Part model, mm, in its own coordinate system. Give positions to 0.01 mm unless a question says otherwise; leave off trailing zeros. Write each loop counter-clockwise with the first axis right and the second up, starting at its lowest first coordinate (ties: lowest second). Pieces come first, ordered by that corner, then holes. Notation, with made-up numbers: M -5,-25.5 L 7,-25.5 A21 ccw 7,6.5 Z; hole C 76.25,-33.5 d1. An arc over 180 degrees is marked long. Use CSV: the item, a comma, the result in double quotes. Start each with the question number.
Item 1: Mould opens along Z. For faces 1 (the flat face through (35, 8, 0)), 2 (the flat face through (35, 8, 4)), 3 (the cylindrical face through (0, 8, 2)) say: released by +Z, released by -Z, zero draft, split by the parting line, or undercut.
Item 2: Cut at B-B (z = 2.1). List the corners of the cut face in (x, y), then the cut area to 3 significant figures.
Item 3: Cut at D-D (y = 2.5). List the corners of the cut face in (x, z).
Item 4: Cut at A-A (y = 7.5). List the corners of the cut face in (x, z).
Item 5: Cut at C-C (x = 30). List the corners of the cut face in (y, z).
Item 6: Drill centre lines: line 1 (Y direction, x = 60, z = 1.3); line 2 (X direction, y = 6, z = 0.8); line 3 (X direction, y = 8.75, z = 2.7). Where is each one in solid material? Low to high. Write a range as [from, to].
from build123d import *

# Parameters (mm, degrees)
EXTRUDE_1_DEPTH     = 4
SKETCH_2_R          = 4
SKETCH_2_R_2        = 3
CUT_EXTRUDE_1_DEPTH = 4


with BuildPart() as part:
    # Эскиз1 → Бобышка-Вытянуть1 (new body)
    with BuildSketch(Plane.XY):
        with BuildLine():
            Line((7.483128905, 0), (62.502687585, 0))
            ThreePointArc((62.502687585, 0), (70.002687585, 7.5), (62.502687585, 15))
            Line((62.502687585, 15), (7.483128905, 15))
            ThreePointArc((7.483128905, 15), (-0.016871095, 7.5), (7.483128905, 0))
        make_face()
    extrude(amount=EXTRUDE_1_DEPTH)

    # Эскиз2 → Вырез-Вытянуть1 (cut)
    with BuildSketch(Plane.XY.offset(4)):
        with Locations((8, 7.5)):
            Circle(SKETCH_2_R)
        with Locations((30, 7.5)):
            Circle(SKETCH_2_R_2)
        with Locations((60, 7.5)):
            Circle(SKETCH_2_R_2)
    extrude(amount=-CUT_EXTRUDE_1_DEPTH, mode=Mode.SUBTRACT)


solid = part.part
Worked answers:
1,face 1,"released by -Z"
1,face 2,"released by +Z"
1,face 3,"zero draft"
2,outline,"M 7.48,0 L 62.5,0 A7.5 ccw 62.5,15 L 7.48,15 A7.5 ccw Z; hole C 8,7.5 d8; hole C 30,7.5 d6; hole C 60,7.5 d6"
2,area,"895 mm^2"
3,outline,"M 1.89,0 L 68.09,0 L 68.09,4 L 1.89,4 Z"
4,outline,"M -0.02,0 L 4,0 L 4,4 L -0.02,4 Z; M 12,0 L 27,0 L 27,4 L 12,4 Z; M 33,0 L 57,0 L 57,4 L 33,4 Z; M 63,0 L 70,0 L 70,4 L 63,4 Z"
5,outline,"M 0,0 L 4.5,0 L 4.5,4 L 0,4 Z; M 10.5,0 L 15,0 L 15,4 L 10.5,4 Z"
6,line 1,"y = [0, 4.5], [10.5, 15]"
6,line 2,"x = [0.13, 4.29], [11.71, 27.4], [32.6, 57.4], [62.6, 69.85]"
6,line 3,"x = [0.09, 4.2], [11.8, 27.27], [32.73, 57.27], [62.73, 69.9]"
